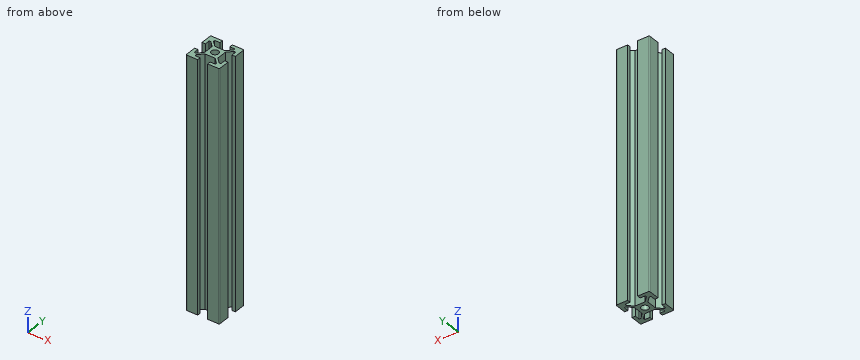
```python
from build123d import *

# Parameters (mm, degrees)
SKETCH1_R           = 2.15
BOSS_EXTRUDE1_DEPTH = 150


with BuildPart() as part:
    # Sketch1 → Boss-Extrude1 (new body)
    with BuildSketch(Plane.XY):
        with BuildLine():
            Line((-3, 10), (-9.5, 10))
            ThreePointArc((-9.5, 10), (-9.853553391, 9.853553391), (-10, 9.5))
            Line((-10, 9.5), (-10, 3))
            Line((-10, 3), (-8, 3))
            Line((-8, 3), (-8, 6.080761184))
            Line((-8, 6.080761184), (-7, 6.080761184))
            Line((-7, 6.080761184), (-4, 3.080761184))
            Line((-4, 3.080761184), (-4, -3.080761184))
            Line((-4, -3.080761184), (-7, -6.080761184))
            Line((-7, -6.080761184), (-8, -6.080761184))
            Line((-8, -6.080761184), (-8, -3))
            Line((-8, -3), (-10, -3))
            Line((-10, -3), (-10, -9.5))
            ThreePointArc((-10, -9.5), (-9.853553391, -9.853553391), (-9.5, -10))
            Line((-9.5, -10), (-3, -10))
            Line((-3, -10), (-3, -8))
            Line((-3, -8), (-6.080761184, -8))
            Line((-6.080761184, -8), (-6.080761184, -7))
            Line((-6.080761184, -7), (-3.080761184, -4))
            Line((-3.080761184, -4), (3.080761184, -4))
            Line((3.080761184, -4), (6.080761184, -7))
            Line((6.080761184, -7), (6.080761184, -8))
            Line((6.080761184, -8), (3, -8))
            Line((3, -8), (3, -10))
            Line((3, -10), (9.5, -10))
            ThreePointArc((9.5, -10), (9.853553391, -9.853553391), (10, -9.5))
            Line((10, -9.5), (10, -3))
            Line((10, -3), (8, -3))
            Line((8, -3), (8, -6.080761184))
            Line((8, -6.080761184), (7, -6.080761184))
            Line((7, -6.080761184), (4, -3.080761184))
            Line((4, -3.080761184), (4, 3.080761184))
            Line((4, 3.080761184), (7, 6.080761184))
            Line((7, 6.080761184), (8, 6.080761184))
            Line((8, 6.080761184), (8, 3))
            Line((8, 3), (10, 3))
            Line((10, 3), (10, 9.5))
            ThreePointArc((10, 9.5), (9.853553391, 9.853553391), (9.5, 10))
            Line((9.5, 10), (3, 10))
            Line((3, 10), (3, 8))
            Line((3, 8), (6.080761184, 8))
            Line((6.080761184, 8), (6.080761184, 7))
            Line((6.080761184, 7), (3.080761184, 4))
            Line((3.080761184, 4), (-3.080761184, 4))
            Line((-3.080761184, 4), (-6.080761184, 7))
            Line((-6.080761184, 7), (-6.080761184, 8))
            Line((-6.080761184, 8), (-3, 8))
            Line((-3, 8), (-3, 10))
        make_face()
        Circle(SKETCH1_R, mode=Mode.SUBTRACT)
    extrude(amount=BOSS_EXTRUDE1_DEPTH)


solid = part.part
```
Can you work these out from the model? Positions are in its coordinate system, mm. Coordinates: 2 decimals unless noted, no trailing zeros. Loops run counter-clockwise (first coordinate to the right, second up) from the corner with the lowest first, then second, coordinate; pieces in that order, holes last. Notation, with made-up numbers: M -24.5,-2.75 L -4.5,-2.75 A21 ccw -4.5,15.25 Z; hole C 23,57.25 d1. An arc over 180 degrees is marked long. Put each result on its own line as item: value. Start each with the question number.
(1) Imagine slicing it at A-A on y = 0. List the corners of the cut face in (x, z) for me.
(2) I need wall thicknesses on probe 1 along Y at (x, z) = (0, 96.5); probe 2 along X at (y, z) = (3.25, 134); probe 3 along Y at (x, z) = (2.25, 15). Which ranges of each line are inside material? Lowest first, please.
(3) Will these pins go through, and if not, where does the flat tip stop? pin 1 Ø2.5 at (x, y) = (0, 0) entering from -Z; pin 2 Ø2 at (y, z) = (1.5, 62) entering from +X.
Worked answers:
1. outline: M -4,0 L -2.15,0 L -2.15,150 L -4,150 Z; M 2.15,0 L 4,0 L 4,150 L 2.15,150 Z
2. probe 1: y = -4 to -2.15, 2.15 to 4
2. probe 2: x = -10 to -8, -4.17 to 4.17, 8 to 10
2. probe 3: y = -4 to 4
3. pin 1: passes through
3. pin 2: stops at x = 4
